```python
from build123d import *

# Parameters (mm, degrees)
SKETCH1_W           = 609.6
SKETCH1_H           = 38.1
BOSS_EXTRUDE1_DEPTH = 6.35
CUT_EXTRUDE1_DEPTH  = 609.6


with BuildPart() as part:
    # Sketch1 → Boss-Extrude1 (new body)
    with BuildSketch(Plane(origin=(0, 0, 0), x_dir=(1, 0, 0), z_dir=(0, 1, 0))):
        Rectangle(SKETCH1_W, SKETCH1_H)
    extrude(amount=BOSS_EXTRUDE1_DEPTH)

    # Sketch2 → Cut-Extrude1 (cut)
    with BuildSketch(Plane.ZY.offset(304.8)):
        Polygon((-10.16, 6.35), (-10.16, 5.55625), (-18.25625, 5.55625), (-18.25625, 0.79375), (-6.35, 0.79375), (-6.35, 2.38125), (6.35, 2.38125), (6.35, 0.79375), (18.25625, 0.79375), (18.25625, 5.55625), (10.16, 5.55625), (10.16, 6.35), align=None)
    extrude(amount=-CUT_EXTRUDE1_DEPTH, mode=Mode.SUBTRACT)


solid = part.part
```
Work out the finished part from the listing and answer in its coordinate system (mm). A direction names the side the tool comes from. Round coordinates to 2 decimals unless told otherwise and drop trailing zeros. Order: outer loops, then holes, each group sorted by start corner. A loop starts at its lowest first (then second) coordinate and runs counter-clockwise, first axis right, second up.
Q1. A cutting plane is placed at A-A, the plane y = 4.25. Determine the outline of the cut face in (x, z), then the cut area to 3 significant figures.
Solution:
outline: (-304.8, -19.05) - (304.8, -19.05) - (304.8, -18.26) - (-304.8, -18.26) - close; (-304.8, 18.26) - (304.8, 18.26) - (304.8, 19.05) - (-304.8, 19.05) - close
area: 968 mm2
Q2. Given pin 1 Ø10 at (x, z) = (-68, -0.5) entering from +Y, flat-ended and moving along its own axis, determine where the tip first touches the part or whether it passes through.
Solution:
pin 1: stops at y = 2.38
Q3. The mould has two halves that part along Z. Classify faces 3 (the flat face through (-4, 0.794, 12)), 4 (the flat face through (-4, 0, 0)): pulls with the +Z half, pulls with the -Z half, needs draft (parallel to the pull), parting line crosses it, or undercut.
Solution:
face 3: undercut
face 4: needs draft
Q4. Find the intervals of material crossed by line 1 along Z through (x, y) = (239, 1.5); line 2 along Z through (x, y) = (216, 5); line 3 along Z through (x, y) = (-46, 5.75), in increasing order.
Solution:
line 1: z = -19.05 to -18.26, -6.35 to 6.35, 18.26 to 19.05
line 2: z = -19.05 to -18.26, 18.26 to 19.05
line 3: z = -19.05 to -10.16, 10.16 to 19.05
Q5. A cutting plane is placed at B-B, the plane x = 70. Determine the outline of the cut face in (y, z), then the cut area to 3 significant figures.
Solution:
outline: (0, -19.05) - (6.35, -19.05) - (6.35, -10.16) - (5.56, -10.16) - (5.56, -18.26) - (0.79, -18.26) - (0.79, -6.35) - (2.38, -6.35) - (2.38, 6.35) - (0.79, 6.35) - (0.79, 18.26) - (5.56, 18.26) - (5.56, 10.16) - (6.35, 10.16) - (6.35, 19.05) - (0, 19.05) - close
area: 72.1 mm2
Q6. A tool of negligible diameter and unlimited length cuts with its end or side. For faces 1 (the flat face through (-4, 0.794, -12)), 2 (the flat face through (-4, 2.381, 0)), from which of +Z, -Z, +X, -X, +Y, -Y can it reach the whole face along a straight path? Write none if from no direction.
Solution:
face 1: +X, -X
face 2: +X, -X, +Y
